from build123d import *

# Parameters (mm, degrees)
F0_W         = 50
F0_H         = 35
F1_DEPTH     = 35
F3_D         = 15.5
F3_DEPTH     = 18
F3_TIP       = 4.6566697975
F5_D         = 15.5
F5_DEPTH     = 18
F5_TIP       = 4.6566697975
F7_D         = 8
F7_DEPTH     = 33
F7_TIP       = 2.4034424761
F8_R         = 10
F8_R_2       = 7.75
F9_DEPTH     = 0.5
F10_R        = 10
F10_R_2      = 7.75
F11_DEPTH    = 0.5
F13_SIZE     = 1
F14_T1_DEPTH = 39.1433659759
F14_T3_DEPTH = 39.1433659759
F14_T5_DEPTH = 55.1433659759
F14_T7_DEPTH = 50.2571417204


# Not quite as in the source:
# - a fillet or chamfer that OpenCascade refuses, or shapes differently, is made with other operations: its cross-section is extruded or revolved along the edge and cut away or added
# - a feature of the source that left no trace in its solid (it failed there, or was rolled back) is left out


with BuildPart() as f1:
    # F0 (on Front) → F1 (new body)
    with BuildSketch(Plane.XZ):
        with Locations((25, 17.5)):
            Rectangle(F0_W, F0_H)
    extrude(amount=F1_DEPTH)

    # F3
    with Locations(Plane.YZ.offset(50)):
        with Locations((-17.5, 17.5)):
            Hole(F3_D / 2, depth=F3_DEPTH)
            with Locations((0, 0, -(F3_DEPTH + F3_TIP / 2))):  # 118° drill point
                Cone(0, F3_D / 2, F3_TIP, mode=Mode.SUBTRACT)

    # F5
    with Locations(Plane.XY.offset(35)):
        with Locations((17.5, -17.5)):
            Hole(F5_D / 2, depth=F5_DEPTH)
            with Locations((0, 0, -(F5_DEPTH + F5_TIP / 2))):  # 118° drill point
                Cone(0, F5_D / 2, F5_TIP, mode=Mode.SUBTRACT)

    # F7
    with Locations(Plane.YZ.offset(50)):
        with Locations((-17.5, 17.5)):
            Hole(F7_D / 2, depth=F7_DEPTH)
            with Locations((0, 0, -(F7_DEPTH + F7_TIP / 2))):  # 118° drill point
                Cone(0, F7_D / 2, F7_TIP, mode=Mode.SUBTRACT)

    # F8 (on face) → F9 (cut)
    with BuildSketch(Plane.YZ.offset(50)):
        with Locations((-17.5, 17.5)):
            Circle(F8_R)
        with Locations((-17.5, 17.5)):
            Circle(F8_R_2, mode=Mode.SUBTRACT)
    extrude(amount=-F9_DEPTH, mode=Mode.SUBTRACT)

    # F10 (on face) → F11 (cut)
    with BuildSketch(Plane.XY.offset(35)):
        with Locations((17.5, -17.5)):
            Circle(F10_R)
        with Locations((17.5, -17.5)):
            Circle(F10_R_2, mode=Mode.SUBTRACT)
    extrude(amount=-F11_DEPTH, mode=Mode.SUBTRACT)

    # F13
    f13_edges = [f1.edges().sort_by_distance(p)[0] for p in [
        (0, 0, 17.5),
        (25, 0, 0),
        (50, 0, 17.5),
        (25, 0, 35),
        (0, -17.5, 0),
        (50, -17.5, 0),
        (25, -35, 0),
    ]]
    chamfer(f13_edges, length=F13_SIZE)

    # F14: chamfer of 1 on 6 edges, made by hand

    # F14_s2 → F14_t1 (cut)
    with BuildSketch(Plane.XZ.offset(-1.571682988)):
        Polygon((0, 34), (1, 35), (0, 35), align=None)
        Polygon((49, 35), (50, 34), (50, 35), align=None)
    extrude(amount=F14_T1_DEPTH, mode=Mode.SUBTRACT)

    # F14_s4 → F14_t3 (cut)
    with BuildSketch(Plane.XY.offset(-1.571682988)):
        Polygon((0, -34), (1, -35), (0, -35), align=None)
        Polygon((49, -35), (50, -34), (50, -35), align=None)
    extrude(amount=F14_T3_DEPTH, mode=Mode.SUBTRACT)

    # F14_s6 → F14_t5 (cut)
    with BuildSketch(Plane.YZ.offset(-2.571682988)):
        Polygon((-34, 35), (-35, 34), (-35, 35), align=None)
    extrude(amount=F14_T5_DEPTH, mode=Mode.SUBTRACT)

    # F14_s8 → F14_t7 (cut)
    with BuildSketch(Plane.YZ.offset(-0.1285708602)):
        Polygon((-34.2928932188, 0.2928932188), (-33.5857864376, 0), (-34, 0), align=None)
    extrude(amount=F14_T7_DEPTH, mode=Mode.SUBTRACT)


solid = f1.part
Can you work these out from the model? Positions are in its coordinate system, mm. A direction names the side the tool comes from. Give positions to 0.01 mm unless a question says otherwise; leave off trailing zeros. One line per question, with ' | ' between items.
Item 1: For faces 5 (the face through (50, -25, 10)), 6 (the face through (25.642, -16.633, 13.595)), 7 (the face through (20, -25, 34.5)), which set-ups out of +Z, -Z, +X, -X, +Y, -Y let a thin tool reach every point of the face, with its end or its side?
Answer block:
face 5: +Z, -Z, +X, +Y, -Y | face 6: +X | face 7: +Z
Item 2: We'd pull the mould along Z, two halves only. Please class faces 1 (the face through (25, 0, 18)), 2 (the face through (40.628, -21.666, 24.035)), 3 (the face through (25, -17, 0)), 4 (the face through (29.89, -18.05, 21.7)): released by +Z, released by -Z, zero draft, split by the parting line, or undercut.
Answer block:
face 1: zero draft | face 2: undercut | face 3: released by -Z | face 4: undercut
Item 3: Please list where these lines run through material, in increasing order: L1, parallel to Y at x = 17.5, z = 21.75; L2, parallel to X at y = -25, z = 11; L3, parallel to X at y = -17.5, z = 27.
Answer block:
L1: y = -35 to -25.25, -9.75 to 0 | L2: x = 0 to 49.5 | L3: x = 0 to 9.75, 25.25 to 49.5
Item 4: I'm going to push flat-ended pins straight in: pin 1 Ø10 at (x, y) = (19, -20.5) entering from +Z; pin 2 Ø5 at (y, z) = (-17.5, 17.5) entering from +X; pin 3 Ø10 at (y, z) = (-19.5, 16.5) entering from +X. Where does each tip first touch, or does it pass through?
Answer block:
pin 1: stops at z = 34.5 | pin 2: stops at x = 13.08 | pin 3: stops at x = 31.69
